The model under review builds one solid part; all positions refer to its coordinate system, in mm. A direction names the side the tool comes from. Coordinates: 2 decimals unless noted, no trailing zeros. Order: outer loops, then holes, each group sorted by start corner. A loop starts at its lowest first (then second) coordinate and runs counter-clockwise, first axis right, second up. Notation, with made-up numbers: M -40,-15 L -25,-15 A25 cw -25,7 Z; hole C 84.25,-22.5 d2. An arc over 180 degrees is marked long. Answer in a Markdown table with one row per item.
from build123d import *

# Parameters (mm, degrees)
SKETCH1_W           = 200
SKETCH1_H           = 100
BOSS_EXTRUDE1_DEPTH = 25
SKETCH2_R           = 6.25
CUT_EXTRUDE1_DEPTH  = 87.5
SKETCH3_R           = 6.25
CUT_EXTRUDE2_DEPTH  = 18.75


with BuildPart() as part:
    # Sketch1 → Boss-Extrude1 (new body)
    with BuildSketch(Plane(origin=(0, 0, 0), x_dir=(1, 0, 0), z_dir=(0, 1, 0))):
        with Locations((17.047695894, 11.5815341)):
            Rectangle(SKETCH1_W, SKETCH1_H)
    extrude(amount=BOSS_EXTRUDE1_DEPTH)

    # Sketch2 → Cut-Extrude1 (cut)
    with BuildSketch(Plane.XY.offset(38.4184659)):
        with Locations((-45.452304106, 12.5)):
            Circle(SKETCH2_R)
        with Locations((79.547695894, 12.5)):
            Circle(SKETCH2_R)
    extrude(amount=-CUT_EXTRUDE1_DEPTH, mode=Mode.SUBTRACT)

    # Sketch3 → Cut-Extrude2 (cut)
    with BuildSketch(Plane(origin=(0, 25, 0), x_dir=(1, 0, 0), z_dir=(0, 1, 0))):
        with Locations(Location((-45.452304106, -13.4184659, 0), (0, 0, 270))):
            Circle(SKETCH3_R)
        with Locations(Location((-45.452304106, 49.0815341, 0), (0, 0, 270))):
            Circle(SKETCH3_R)
        with Locations(Location((79.547695894, 17.8315341, 0), (0, 0, 270))):
            Circle(SKETCH3_R)
    extrude(amount=-CUT_EXTRUDE2_DEPTH, mode=Mode.SUBTRACT)


solid = part.part
(1) Take a section at A-A (z = -5). Write out the cut boundary in (x, y), then the cut area to 3 significant figures.
Report:
| item | result |
|---|---|
| outline | M -82.95,0 L 117.05,0 L 117.05,25 L -82.95,25 Z; hole C -45.45,12.5 d12.5; hole C 79.55,12.5 d12.5 |
| area | 4,750 mm^2 |
(2) Machinability: for faces 4 (the cylindrical face through (-45.178, 15.756, -55.325)), 5 (the flat face through (117.048, 12, -11)), 6 (the cylindrical face through (85.321, 10.106, 10.687)), which of the approach directions +Z, -Z, +X, -X, +Y, -Y give a long, thin tool a straight path to every point of the face, cutting with its end or side? Answer none if there is none.
Report:
| item | result |
|---|---|
| face 4 | +Y |
| face 5 | +Z, -Z, +X, +Y, -Y |
| face 6 | +Z |
(3) Take a section at B-B (y = 15.25). Write out the cut boundary in (x, z), then the cut area to 3 significant figures.
Report:
| item | result |
|---|---|
| outline | M -82.95,-61.58 L 117.05,-61.58 L 117.05,38.42 L 85.16,38.42 L 85.16,-15.08 A6.25 cw 85.16,-20.58 L 85.16,-49.08 L 73.94,-49.08 L 73.94,-20.58 A6.25 cw 73.94,-15.08 L 73.94,38.42 L -39.84,38.42 L -39.84,16.17 A6.25 cw -39.84,10.67 L -39.84,-46.33 A6.25 cw long -51.06,-46.33 L -51.06,10.67 A6.25 cw -51.06,16.17 L -51.06,38.42 L -82.95,38.42 Z |
| area | 18,000 mm^2 |
(4) To check wall thickness, follow line 1 (X direction, y = 12, z = -3.5); line 2 (X direction, y = 18.25, z = 16.5); line 3 (X direction, y = 15.5, z = -51.5). State the ranges of each line that lie inside material, in increasing order. Write a range as [from, to].
Report:
| item | result |
|---|---|
| line 1 | [-82.95, -51.68], [-39.22, 73.32], [85.78, 117.05] |
| line 2 | [-82.95, -50.89], [-40.01, 77.1], [82, 117.05] |
| line 3 | [-82.95, -51.22], [-39.69, 117.05] |
(5) Insertion check: P1, Ø11, axis at x = -45.45, y = 12.5, coming from the +Z side; P2, Ø4, axis at x = 81, y = 10, coming from the +Z side; P3, Ø10, axis at x = -45.45, z = 13.42, coming from the +Y side. Each pin has a flat end and moves straight along its axis. Give the tip position at first contact, or say it passes through.
Report:
| item | result |
|---|---|
| P1 | z = -52.05 |
| P2 | z = -49.08 |
| P3 | y = 6.25 |
(6) The part is to be moulded in two halves that separate along Y. For faces 1 (the cylindrical face through (73.304, 12.775, -36.71)), 2 (the flat face through (16, 12, 38.418)), 3 (the flat face through (16, 0, -12)), say which applies: +Y half, -Y half, draft (parallel to the pull), parting line (faces both ways), or undercut.
Report:
| item | result |
|---|---|
| face 1 | undercut |
| face 2 | draft |
| face 3 | -Y half |
